Input: part model. Units: mm. Frame: model coordinates. A direction names the side the tool comes from. Coordinates: 2 decimals unless noted, no trailing zeros. Write each loop counter-clockwise with the first axis right and the second up, starting at its lowest first coordinate (ties: lowest second). Pieces come first, ordered by that corner, then holes. Notation, with made-up numbers: (31.25, 26.25) - (48.25, 26.25) arc R22 ccw to (48.25, 55.25) - close; hole circle Ø11 at (29, 3.5). An arc over 180 degrees is marked (long way). Put each result on its own line as item: value. Start each with the question number.
1. Cut plane D-D, the plane y = 1.2. Return loops of the section in (x, z).
2. Pull-direction query (X, two-part tool) for faces 4 (the cylindrical face through (-3, 0, 3)), 5 (the flat face through (1.05, 0, 1)), 6 (the cylindrical face through (-1.216, 1.115, 4.173)), 7 (the flat face through (1.3, 0, 0)); classes: released by +X, released by -X, zero draft, split by the parting line, or undercut.
3. Access query for faces 1 (the flat face through (0, 0, 2.5)), 2 (the flat face through (1.3, -1.3, 5.8)), 3 (the flat face through (0, 0, 2.2)). Directions: +Z, -Z, +X, -X, +Y, -Y. A direction counts if a zero-diameter tool reaches every point of the face in a straight line with its end or side. Return the directions, or none.
4. Cut plane A-A, the plane z = 0.55. Return loops of the section in (x, y).
5. Line query: line 1 (Y direction, x = 0, z = 3.3); line 2 (Z direction, x = -0.15, y = -0.8); line 3 (Y direction, x = 0.3, z = 1.25). Output: solid intervals per line, ascending.
6. Cut plane B-B, the plane y = 0. Return loops of the section in (x, z), and give its area (3 significant figures).
7. Pin query (flat end, axial travel): pin 1 (2 mm diameter, centred on y = -1.5, z = 3, fed in from +X); pin 2 (1 mm diameter, centred on x = -0.5, y = -0.5, fed in from -Z); pin 3 (1 mm diameter, centred on y = -2, z = 3, fed in from +X). Return the tip coordinate at first contact, or that it passes through.
from build123d import *

# Parameters (mm, degrees)
SKETCH006_R     = 3
PAD001_DEPTH    = 5.8
SKETCH007_W     = 2.1
SKETCH007_H     = 2.1
POCKET001_DEPTH = 2.2
SKETCH008_R     = 1.65
POCKET002_DEPTH = 3.3


with BuildPart() as part:
    # Sketch006 → Pad001 (new body)
    with BuildSketch(Plane.XY):
        Circle(SKETCH006_R)
    extrude(amount=PAD001_DEPTH)

    # Sketch007 → Pocket001 (cut)
    with BuildSketch(Plane.XY):
        Rectangle(SKETCH007_W, SKETCH007_H)
    extrude(amount=POCKET001_DEPTH, mode=Mode.SUBTRACT)

    # Sketch008 (on Face3 of Pocket001) → Pocket002 (cut)
    with BuildSketch(Plane.XY.offset(5.8)):
        Circle(SKETCH008_R)
    extrude(amount=-POCKET002_DEPTH, mode=Mode.SUBTRACT)


solid = part.part
Report:
1. outline: (-2.75, 0) - (2.75, 0) - (2.75, 5.8) - (1.13, 5.8) - (1.13, 2.5) - (-1.13, 2.5) - (-1.13, 5.8) - (-2.75, 5.8) - close
2. face 4: split by the parting line
2. face 5: undercut
2. face 6: undercut
2. face 7: zero draft
3. face 1: +Z
3. face 2: +Z, +X, -X, +Y, -Y
3. face 3: -Z
4. outline: circle Ø6 at (0, 0); hole (-1.05, -1.05) - (1.05, -1.05) - (1.05, 1.05) - (-1.05, 1.05) - close
5. line 1: y = -3 to -1.65, 1.65 to 3
5. line 2: z = 2.2 to 2.5
5. line 3: y = -2.98 to -1.05, 1.05 to 2.98
6. outline: (-3, 0) - (-1.05, 0) - (-1.05, 2.2) - (1.05, 2.2) - (1.05, 0) - (3, 0) - (3, 5.8) - (1.65, 5.8) - (1.65, 2.5) - (-1.65, 2.5) - (-1.65, 5.8) - (-3, 5.8) - close
6. area: 19.3 mm^2
7. pin 1: stops at x = 2.96
7. pin 2: stops at z = 2.2
7. pin 3: stops at x = 2.6
